Study the drawing (mm; zero at the part's minimum x, y, z) and answer. A direction names the side the tool comes from. Round coordinates to 2 decimals unless told otherwise and drop trailing zeros. Order: outer loops, then holes, each group sorted by start corner. A loop starts at its lowest first (then second) coordinate and runs counter-clockwise, first axis right, second up. Notation, with made-up numbers: (-26, 77.5) - (8, 77.5) arc R15 ccw to (8, 92.5) - close; hole circle Ø8 at (-39, 31.25). An arc over 180 degrees is marked (long way). Put each result on its own line as item: value. Start each with the question number.
Q1. Which of the six approach directions +Z, -Z, +X, -X, +Y, -Y give full straight-line access (tool end or side, diameter ignored) to the marked faces 5 and 6?
Q2. For a pull along Y with two mould halves and no side action, classify the marked faces 1, 2, 3 and 4 as pulls with the +Y half, pulls with the -Y half, needs draft (parallel to the pull), parting line crosses it, or undercut.
Q3. Section C-C on z = 17.78 is taken. State how many separate pieces and enclosed holes the cut face has, then the cut area to 3 significant figures.
Q4. Section B-B on y = 8 is taken. Give the vertices of the cut face in (x, z) (1 decimal).
Q5. Find the intervals of material crossed by line 1 along X through (y, z) = (27.5, 7.5) (1 decimal); line 2 along Y through (x, z) = (5.5, 13.25) (1 decimal); line 3 along Y through (x, z) = (3, 4.75) (1 decimal), in increasing order. Write a range as from..to.
Q6. Section A-A on x = 17.78 is taken. Give the vertices of the cut face in (y, z), then the cut area to 3 significant figures.
Q7. Section D-D on z = 12 is taken. Give the vertices of the cut face in (x, y), then the cut area to 3 significant figures.
Q8. Each of these flat-tipped pins is pushed along its axis until it touches: pin 1 Ø2.5 at (y, z) = (25.18, 17.78) entering from +X; pin 2 Ø1.7 at (x, y) = (17.78, 21.37) entering from -Z. Where does it stop, or does it pass through?
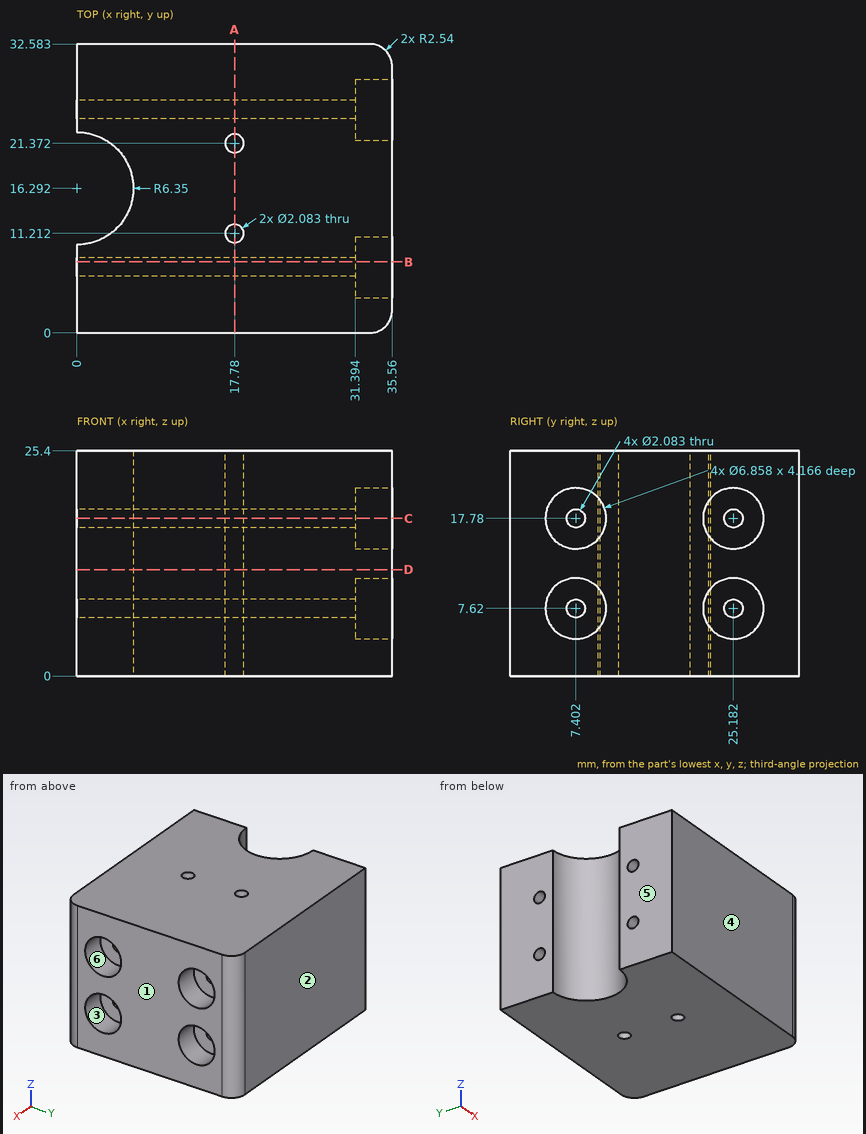
Findings:
1. face 5: +Z, -Z, -X, +Y, -Y
1. face 6: +X
2. face 1: needs draft
2. face 2: pulls with the +Y half
2. face 3: undercut
2. face 4: pulls with the -Y half
3. separate pieces: 3
3. enclosed holes: 2
3. area: 898 mm2
4. outline: (0, 0) - (35.6, 0) - (35.6, 4.2) - (31.4, 4.2) - (31.4, 6.8) - (0, 6.8) - close; (0, 8.5) - (31.4, 8.5) - (31.4, 11) - (35.6, 11) - (35.6, 14.4) - (31.4, 14.4) - (31.4, 16.9) - (0, 16.9) - close; (0, 18.6) - (31.4, 18.6) - (31.4, 21.2) - (35.6, 21.2) - (35.6, 25.4) - (0, 25.4) - close
5. line 1: 0..31.4
5. line 2: 0..13.1, 19.5..32.6
5. line 3: 0..10.7, 21.9..32.6
6. outline: (0, 0) - (10.17, 0) - (10.17, 25.4) - (0, 25.4) - close; (12.25, 0) - (20.33, 0) - (20.33, 25.4) - (12.25, 25.4) - close; (22.41, 0) - (32.58, 0) - (32.58, 25.4) - (22.41, 25.4) - close; hole circle Ø2.08 at (7.4, 7.62); hole circle Ø2.08 at (7.4, 17.78); hole circle Ø2.08 at (25.18, 7.62); hole circle Ø2.08 at (25.18, 17.78)
6. area: 708 mm2
7. outline: (0, 0) - (33.02, 0) arc R2.54 ccw to (35.56, 2.54) - (35.56, 30.04) arc R2.54 ccw to (33.02, 32.58) - (0, 32.58) - (0, 22.64) arc R6.35 cw to (0, 9.94) - close; hole circle Ø2.08 at (17.78, 11.21); hole circle Ø2.08 at (17.78, 21.37)
7. area: 1,090 mm2
8. pin 1: x = 31.39
8. pin 2: through
